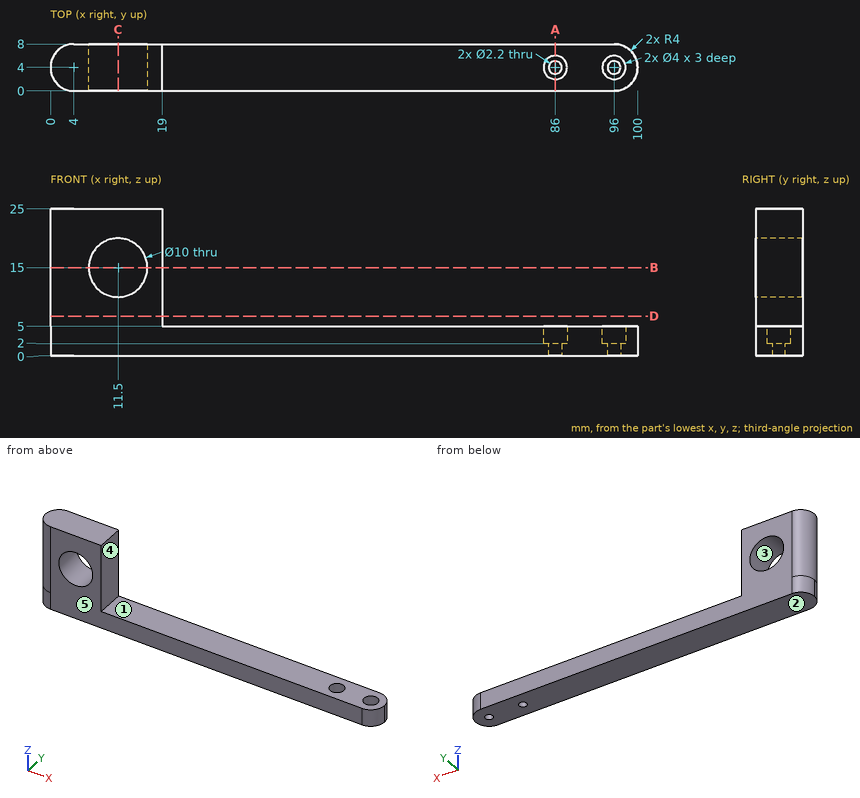
The drawing under review shows one solid part. Ordinate dimensions are in mm from its lowest x, y, z. A direction names the side the tool comes from. Coordinates: 2 decimals unless noted, no trailing zeros. Order: outer loops, then holes, each group sorted by start corner. A loop starts at its lowest first (then second) coordinate and runs counter-clockwise, first axis right, second up. Notation, with made-up numbers: (74, 61) - (101, 61) arc R10 ccw to (101, 70) - close; hole circle Ø1 at (54.25, -3.75). An arc over 180 degrees is marked (long way). Put each result on its own line as item: value.
1) Take a section at C-C, the plane x = 11.5. Give the boundary of the cut face in (y, z), and give its area (3 significant figures).
Response values:
outline: (0, 0) - (8, 0) - (8, 10) - (0, 10) - close; (0, 20) - (8, 20) - (8, 25) - (0, 25) - close
area: 120 mm²
2) Insertion check: P1, Ø3, axis at x = 96, y = 4, coming from the +Z side; P2, Ø4.5, axis at x = 85.5, y = 3, coming from the +Z side; P3, Ø1, axis at y = 6, z = 18.5, coming from the +X side. Each pin has a flat end and moves straight along its axis. Give the tip position at first contact, or say it passes through.
Response values:
P1: stops at z = 2
P2: stops at z = 5
P3: stops at x = 19
3) Take a section at A-A, the plane x = 86. Give the boundary of the cut face in (y, z).
Response values:
outline: (0, 0) - (2.9, 0) - (2.9, 2) - (2, 2) - (2, 5) - (0, 5) - close; (5.1, 0) - (8, 0) - (8, 5) - (6, 5) - (6, 2) - (5.1, 2) - close
4) Take a section at D-D, the plane z = 6.75. Give the boundary of the cut face in (x, y), and give its area (3 significant figures).
Response values:
outline: (4, 0) - (19, 0) - (19, 8) - (4, 8) arc R4 ccw to start
area: 145 mm²
5) The part is to be moulded in two halves that separate along X. For the marked faces 3, 4 and 5, say which applies: released by +X, released by -X, zero draft, split by the parting line, or undercut.
Response values:
face 3: undercut
face 4: released by +X
face 5: zero draft
6) Wall thickness on L1, parallel to X at y = 4.5, z = 4; L2, parallel to Y at x = 96, z = 0.4; L3, parallel to Y at x = 86, z = 2.75: over which ranges is each line inside the solid? List them lowest first. Write a range as from..to.
Response values:
L1: x = 0.03..84.06, 87.94..94.06, 97.94..99.97
L2: y = 0..2.9, 5.1..8
L3: y = 0..2, 6..8
7) Take a section at B-B, the plane z = 15. Give the boundary of the cut face in (x, y).
Response values:
outline: (4, 0) - (6.5, 0) - (6.5, 8) - (4, 8) arc R4 ccw to start; (16.5, 0) - (19, 0) - (19, 8) - (16.5, 8) - close
8) Tool access review of the marked faces 1 and 2: name each direction out of +Z, -Z, +X, -X, +Y, -Y from which nothing blocks a thin tool from reaching the whole face with its end or side.
Response values:
face 1: +Z, +X, +Y, -Y
face 2: -Z, +X, -X, +Y, -Y
